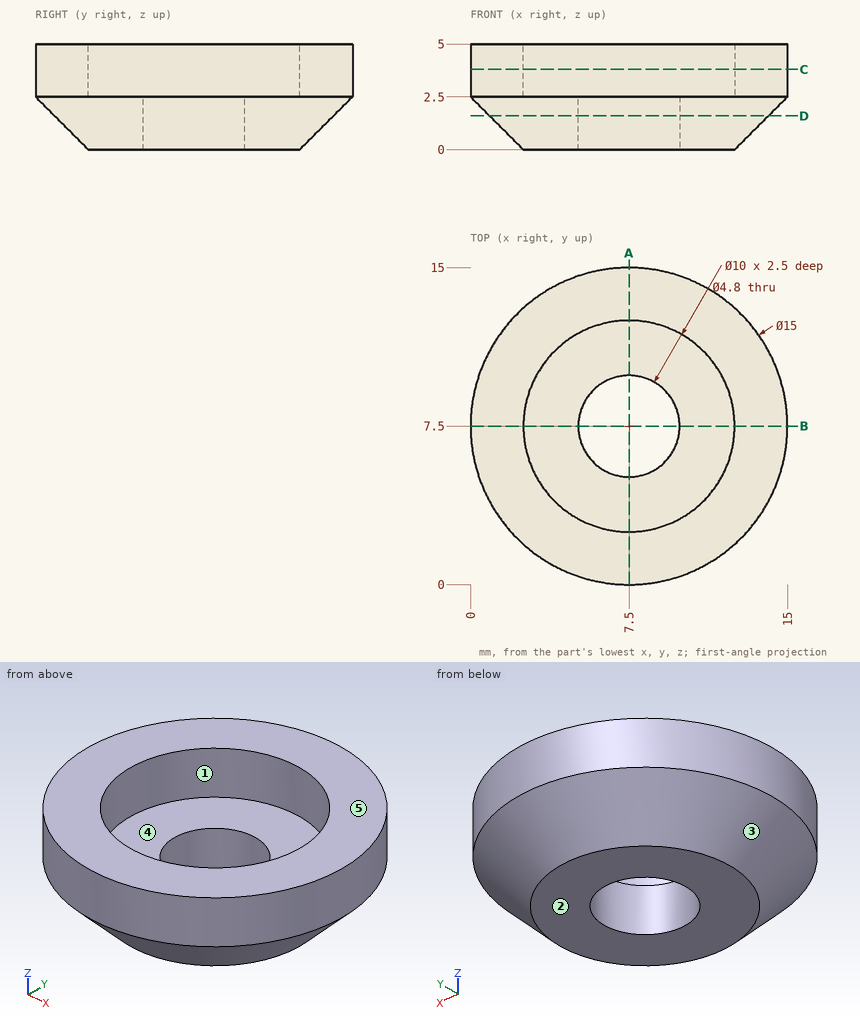
The figure shows three views and two pictorial views of one solid part (mm, origin at its lowest corner). Answer the questions. A direction names the side the tool comes from. Round coordinates to 2 decimals unless told otherwise and drop trailing zeros. Write each loop counter-clockwise with the first axis right and the second up, starting at its lowest first coordinate (ties: lowest second). Pieces come first, ordered by that corner, then holes. Notation, with made-up numbers: (25, 58.5) - (43, 58.5) arc R22 ccw to (43, 82.5) - close; hole circle Ø11 at (43.25, 84). An arc over 180 degrees is marked (long way). Use one line per item in the form item = value. Start each with the question number.
Item 1: A cutting plane is placed at C-C (z = 3.8). Write down the section's boundary in (x, y).
Item 2: Determine the mould class of the marked faces 1, 2 and 3 for opening direction X: +X half, -X half, draft (parallel to the pull), parting line (faces both ways), or undercut.
Item 3: A cutting plane is placed at A-A (x = 7.5). Write down the section's boundary in (y, z), plus the area to 4 significant figures.
Item 4: Find the intervals of material crossed by line 1 (Y direction, x = 7.5, z = 4.2); line 2 (Y direction, x = 6, z = 1.9); line 3 (X direction, y = 8.25, z = 3.85), in increasing order. Write a range as [from, to].
Item 5: A tool of negligible diameter and unlimited length cuts with its end or side. For the marked faces 4 and 5, from which of +Z, -Z, +X, -X, +Y, -Y can it reach the whole face along a straight path? Write none if from no direction.
Item 6: A cutting plane is placed at D-D (z = 1.6). Write down the section's boundary in (x, y), plus the area to 3 significant figures.
Item 7: Flat-ended cylindrical pins translate along their axes: pin 1 Ø1.5 at (y, z) = (4.5, 1) entering from -X; pin 2 Ø1.5 at (y, z) = (9, 3) entering from +X; pin 3 Ø6 at (x, y) = (7.5, 7.5) entering from +Z. Find the tip coordinate at first contact, or state that the pin passes through.
The answers:
q1.outline = circle Ø15 at (7.5, 7.5); hole circle Ø10 at (7.5, 7.5)
q2.face_1 = undercut
q2.face_2 = draft
q2.face_3 = parting line
q3.outline = (0, 2.5) - (2.5, 0) - (5.1, 0) - (5.1, 2.5) - (2.5, 2.5) - (2.5, 5) - (0, 5) - close; (9.9, 0) - (12.5, 0) - (15, 2.5) - (15, 5) - (12.5, 5) - (12.5, 2.5) - (9.9, 2.5) - close
q3.area = 31.75 mm^2
q4.line_1 = [0, 2.5], [12.5, 15]
q4.line_2 = [0.77, 5.63], [9.37, 14.23]
q4.line_3 = [0.04, 2.56], [12.44, 14.96]
q5.face_4 = +Z
q5.face_5 = +Z, +X, -X, +Y, -Y
q6.outline = circle Ø13.2 at (7.5, 7.5); hole circle Ø4.8 at (7.5, 7.5)
q6.area = 119 mm^2
q7.pin_1 = 1.38
q7.pin_2 = 14.96
q7.pin_3 = 2.5
